Model file for the job. Use its own axes, mm. A direction names the side the tool comes from. Round coordinates to 2 decimals unless told otherwise and drop trailing zeros. Loops run counter-clockwise (first coordinate to the right, second up) from the corner with the lowest first, then second, coordinate; pieces in that order, holes last. Notation, with made-up numbers: M -33,68 L -7,68 A24 ccw -7,88 Z; hole C -14.5,-10 d8. An arc over 180 degrees is marked long. Use a Markdown table: item, result. Add a question column.
Q1. Cut at B-B (z = 29). Give the cut face in (x, y), plus the area to 3 significant figures.
Q2. Tool access for faces 1 (the face through (-0.95, 0, 30)), 2 (the face through (0, 0, 18.2)), 3 (the face through (5, -4, 15)), 4 (the face through (-5, -4, 15)): list every direction of +Z, -Z, +X, -X, +Y, -Y with a clear straight run to the whole face (end or side of a thin tool).
Q3. Cut at A-A (x = 0). Give the cut face in (y, z).
Q4. Cut at C-C (z = 11.5). Give the cut face in (x, y), plus the area to 3 significant figures.
Q5. Pin check, flat tips, straight feed: pin 1 (1.5 mm diameter, centred on x = -4.5, z = 13, fed in from +Y); pin 2 (2 mm diameter, centred on x = -3.5, y = 1, fed in from +Z); pin 3 (1.5 mm diameter, centred on x = -1, y = 0, fed in from -Z). Stop position of each tip, or through.
Q6. Probe line 1 (Z direction, x = -4.75, y = 3.5); line 2 (Z direction, x = 2.25, y = 0.75); line 3 (Y direction, x = 3.7, z = -0.65). List the from-to ranges inside material, lowest first. Write a range as from..to.
from build123d import *

# Parameters (mm, degrees)
SALIENTE_EXTRUIR1_DEPTH  = 15
SALIENTE_EXTRUIR2_DEPTH  = 0.8
CROQUIS3_R               = 1.5
SALIENTE_EXTRUIR3_DEPTH  = 2.4
SALIENTE_EXTRUIR4_DEPTH  = 0.8
CROQUIS5_R               = 1.5
SALIENTE_EXTRUIR5_DEPTH  = 4.27
SALIENTE_EXTRUIR6_DEPTH  = 0.8
CROQUIS7_R               = 2
SALIENTE_EXTRUIR7_DEPTH  = 1
CROQUIS8_R               = 1.5
SALIENTE_EXTRUIR8_DEPTH  = 9.2
CORTAR_EXTRUIR1_START    = -9
CORTAR_EXTRUIR1_DEPTH    = 9
CROQUIS1_3_R             = 2.5
SALIENTE_EXTRUIR9_DEPTH  = 1
CROQUIS1_4_W             = 0.3
CROQUIS1_4_H             = 1.5
SALIENTE_EXTRUIR10_DEPTH = 1.3
CORTAR_EXTRUIR2_REACH    = 37.993
CROQUIS10_R              = 0.35


with BuildPart() as part:
    # Croquis1 → Saliente-Extruir1 (new body)
    with BuildSketch(Plane.XY):
        with BuildLine():
            Line((3.31662479, 5), (-3.31662479, 5))
            ThreePointArc((-3.31662479, 5), (-6, 0), (-3.31662479, -5))
            Line((-3.31662479, -5), (3.31662479, -5))
            ThreePointArc((3.31662479, -5), (6, 0), (3.31662479, 5))
        make_face()
    extrude(amount=SALIENTE_EXTRUIR1_DEPTH)

    # Croquis2 → Saliente-Extruir2 (add)
    with BuildSketch(Plane.XY.offset(15)):
        with BuildLine():
            Line((-5.5, -5), (5.5, -5))
            ThreePointArc((5.5, -5), (5.853553391, -4.853553391), (6, -4.5))
            Line((6, -4.5), (6, 4.5))
            ThreePointArc((6, 4.5), (5.853553391, 4.853553391), (5.5, 5))
            Line((5.5, 5), (-5.5, 5))
            ThreePointArc((-5.5, 5), (-5.853553391, 4.853553391), (-6, 4.5))
            Line((-6, 4.5), (-6, -4.5))
            ThreePointArc((-6, -4.5), (-5.853553391, -4.853553391), (-5.5, -5))
        make_face()
    extrude(amount=SALIENTE_EXTRUIR2_DEPTH)

    # Croquis3 → Saliente-Extruir3 (add)
    with BuildSketch(Plane.XY.offset(15.8)):
        with Locations(Location((-3.853553391, -3.195226195, 0), (0, 0, 180))):
            Circle(CROQUIS3_R)
        with Locations(Location((4, 3.316654392, 0), (0, 0, 180))):
            Circle(CROQUIS3_R)
    extrude(amount=SALIENTE_EXTRUIR3_DEPTH)

    # Croquis4 → Saliente-Extruir4 (add)
    with BuildSketch(Plane.XY.offset(18.2)):
        with BuildLine():
            Line((5.5, 5), (-5.5, 5))
            ThreePointArc((-5.5, 5), (-5.853553391, 4.853553391), (-6, 4.5))
            Line((-6, 4.5), (-6, -4.5))
            ThreePointArc((-6, -4.5), (-5.853553391, -4.853553391), (-5.5, -5))
            Line((-5.5, -5), (5.5, -5))
            ThreePointArc((5.5, -5), (5.853553391, -4.853553391), (6, -4.5))
            Line((6, -4.5), (6, 4.5))
            ThreePointArc((6, 4.5), (5.853553391, 4.853553391), (5.5, 5))
        make_face()
    extrude(amount=SALIENTE_EXTRUIR4_DEPTH)

    # Croquis5 → Saliente-Extruir5 (add)
    with BuildSketch(Plane.XY.offset(19)):
        with Locations(Location((4, 3.316654392, 0), (0, 0, 180))):
            Circle(CROQUIS5_R)
        with Locations(Location((-3.853553391, -3.195226195, 0), (0, 0, 180))):
            Circle(CROQUIS5_R)
    extrude(amount=SALIENTE_EXTRUIR5_DEPTH)

    # Croquis6 → Saliente-Extruir6 (add)
    with BuildSketch(Plane.XY.offset(23.27)):
        with BuildLine():
            Line((5.5, 5), (-5.5, 5))
            ThreePointArc((-5.5, 5), (-5.853553391, 4.853553391), (-6, 4.5))
            Line((-6, 4.5), (-6, -4.5))
            ThreePointArc((-6, -4.5), (-5.853553391, -4.853553391), (-5.5, -5))
            Line((-5.5, -5), (5.5, -5))
            ThreePointArc((5.5, -5), (5.853553391, -4.853553391), (6, -4.5))
            Line((6, -4.5), (6, 4.5))
            ThreePointArc((6, 4.5), (5.853553391, 4.853553391), (5.5, 5))
        make_face()
    extrude(amount=SALIENTE_EXTRUIR6_DEPTH)

    # Croquis7 → Saliente-Extruir7 (add)
    with BuildSketch(Plane.XY.offset(24.07)):
        Circle(CROQUIS7_R)
    extrude(amount=SALIENTE_EXTRUIR7_DEPTH)

    # Croquis8 → Saliente-Extruir8 (add)
    with BuildSketch(Plane.XY.offset(25.07)):
        Circle(CROQUIS8_R)
    extrude(amount=SALIENTE_EXTRUIR8_DEPTH)

    # Croquis9 → Cortar-Extruir1 (cut)
    with BuildSketch(Plane.XY.offset(34.27).offset(CORTAR_EXTRUIR1_START)):
        with BuildLine():
            Line((-0.95, -1.160818677), (-0.95, 1.160818677))
            ThreePointArc((-0.95, 1.160818677), (-1.5, 0), (-0.95, -1.160818677))
        make_face()
    extrude(amount=CORTAR_EXTRUIR1_DEPTH, mode=Mode.SUBTRACT)

    # Croquis1_3 → Saliente-Extruir9 (add)
    with BuildSketch(Plane.XY):
        Circle(CROQUIS1_3_R)
    extrude(amount=-SALIENTE_EXTRUIR9_DEPTH)

    # Croquis1_4 → Saliente-Extruir10 (add)
    with BuildSketch(Plane.XY):
        with Locations((-3.65, 0)):
            Rectangle(CROQUIS1_4_W, CROQUIS1_4_H)
    saliente_extruir10 = extrude(amount=-SALIENTE_EXTRUIR10_DEPTH)

    # Croquis10 → Cortar-Extruir2 (cut, up to next)
    with BuildSketch(Plane.ZY.offset(3.8), mode=Mode.PRIVATE) as cortar_extruir2_sk1:
        with Locations((-0.65, 0)):
            Circle(CROQUIS10_R)
    cortar_extruir2_tool1 = extrude(cortar_extruir2_sk1.sketch, amount=-CORTAR_EXTRUIR2_REACH, mode=Mode.PRIVATE) & part.part
    cortar_extruir2 = cortar_extruir2_tool1.solids().sort_by_distance((-3.8, 0, -0.65))[0]
    add(cortar_extruir2, mode=Mode.SUBTRACT)

    # Simetr_a1: Saliente-Extruir10, Cortar-Extruir2 across plane
    add(saliente_extruir10.mirror(Plane(origin=(0, 0, 0), x_dir=(0, 0, 1), z_dir=(1, 0, 0))))
    add(cortar_extruir2.mirror(Plane(origin=(0, 0, 0), x_dir=(0, 0, 1), z_dir=(1, 0, 0))), mode=Mode.SUBTRACT)


solid = part.part
Checked values:
| question | item | result |
|---|---|---|
| 1 | outline | M -0.95,-1.16 A1.5 ccw long -0.95,1.16 Z |
| 1 | area | 6.18 mm^2 |
| 2 | face 1 | +Z, -X, +Y, -Y |
| 2 | face 2 | none |
| 2 | face 3 | -Z, +X, -Y |
| 2 | face 4 | -Z, -X, -Y |
| 3 | outline | M -5,0 L -2.5,0 L -2.5,-1 L 2.5,-1 L 2.5,0 L 5,0 L 5,15.8 L -5,15.8 Z; M -5,18.2 L 5,18.2 L 5,19 L -5,19 Z; M -5,23.27 L 5,23.27 L 5,24.07 L 2,24.07 L 2,25.07 L 1.5,25.07 L 1.5,34.27 L -1.5,34.27 L -1.5,25.07 L -2,25.07 L -2,24.07 L -5,24.07 Z |
| 4 | outline | M -3.32,-5 L 3.32,-5 A6 ccw 3.32,5 L -3.32,5 A6 ccw Z |
| 4 | area | 104 mm^2 |
| 5 | pin 1 | stops at y = 4.68 |
| 5 | pin 2 | stops at z = 24.07 |
| 5 | pin 3 | stops at z = -1 |
| 6 | line 1 | z = 0..15.8, 18.2..19, 23.27..24.07 |
| 6 | line 2 | z = -1..15.8, 18.2..19, 23.27..24.07 |
| 6 | line 3 | y = -0.75..-0.35, 0.35..0.75 |
